Design review of the part built by this model. Coordinates are the model's own, in mm. Face numbers are marked on the shaded views. A direction names the side the tool comes from. Give positions to 0.01 mm unless a question says otherwise; leave off trailing zeros. Write each loop counter-clockwise with the first axis right and the second up, starting at its lowest first coordinate (ties: lowest second). Pieces come first, ordered by that corner, then holes. Notation, with made-up numbers: (78.25, 45.5) -> (134.25, 45.5) arc R22 ccw to (134.25, 77.5) -> close; hole circle Ø5 at (78.5, -19). An arc over 180 degrees is marked (long way). Answer as a JSON object with one key per item and string values.
Autodesk Inventor part; units mm, degrees
ref_plane "YZ Plane" through (0, 0, 0) normal (1, 0, 0) x (0, 1, 0)
ref_plane "XZ Plane" through (0, 0, 0) normal (0, 1, 0) x (-1, 0, 0)
ref_plane "XY Plane" through (0, 0, 0) normal (0, 0, 1) x (1, 0, 0)
sketch "Skizze1" plane through (0, 0, 0) normal (0, 0, 1) x (1, 0, 0)
  circle A0 centre (0, 0) radius 4
  line L0 (2.3094, 4) -> (9.9282, 4)
  line L1 (9.9282, 4) -> (9.9282, -4)
  line L2 (9.9282, -4) -> (6.9282, -4)
  line L3 (6.9282, -4) -> (2.3094, 4)
  line L4 (0, -4) -> (6.9282, -4)
  line L5 (2.3094, 4) -> (0, 4)
  dimension "d0" = 8
  dimension "d2" = 60
  dimension "d10" = 3
extrude "Extrusion1" add sketch "Skizze1" along normal blind 3
extrude "Extrusion2" add sketch "Skizze1" against normal blind 3 contours L3 L0 L1 L2
sketch "Skizze2" plane through (0, 0, 3) normal (0, 0, 1) x (1, 0, 0)
  line L0 (2.3094, 4) -> (9.9282, 4)
  line L1 (9.9282, 4) -> (9.9282, -4)
  line L2 (9.9282, -4) -> (6.9282, -4)
  line L3 (6.9282, -4) -> (2.3094, 4)
  line L4 (6.9282, -4) -> (9.9282, -4)
  line L5 (9.9282, -4) -> (9.9282, 4)
  line L6 (9.9282, 4) -> (6.9282, 4)
  line L7 (6.9282, 4) -> (6.9282, -4)
extrude "Extrusion3" add sketch "Skizze2" along normal blind 6.5 contours L0 L1 L2 L7
mirror "Spiegeln1" about plane through (8.4282, 0, 9.5) normal (0, 0, 1)
sketch "Skizze4" plane through (0, 0, 3) normal (0, 0, 1) x (1, 0, 0)
  line L0 (6.9282, -4) -> (6.9282, 4)
  line L1 (6.9282, 4) -> (0, 4)
  arc A0 (0, 4) -> (0, -4) centre (0, 0) ccw
  line L2 (0, -4) -> (6.9282, -4)
  line L3 (2.3094, 4) -> (9.9282, 4)
  line L4 (9.9282, 4) -> (9.9282, -4)
  line L5 (9.9282, -4) -> (6.9282, -4)
  line L6 (6.9282, -4) -> (2.3094, 4)
  line L7 (-4, 0) -> (-4, -8)
  line L8 (0, 0) -> (0, -8) construction
  line L9 (9.9282, -4) -> (2.773, -10.8828)
  arc A1 (-4, -8) -> (2.773, -10.8828) centre (0, -8) ccw
  arc A2 (0, 4) -> (-4, 0) centre (0, 0) ccw
  line L10 (0, 4) -> (9.9282, 4)
  line L11 (9.9282, -4) -> (9.9282, 4)
  dimension "d18" = 8
extrude "Extrusion4" [suppressed]
extrude "Extrusion5" add sketch "Skizze4" along normal blind 3
sketch "Skizze5" plane through (0, 0, -3) normal (0, 0, -1) x (-1, 0, 0)
  line L0 (-2.3094, 4) -> (-6.9282, -4)
  line L1 (0, -4) -> (-6.9282, -4)
  arc A0 (0, -4) -> (0, 4) centre (0, 0) ccw
  line L2 (-2.3094, 4) -> (0, 4)
  line L3 (0, -4) -> (-9.9282, -4)
  line L4 (-2.773, -10.8828) -> (-9.9282, -4)
  arc A1 (-2.773, -10.8828) -> (4, -8) centre (0, -8) ccw
  line L5 (4, 0) -> (4, -8)
  arc A2 (0, -4) -> (4, 0) centre (0, 0) ccw
hole "Bohrung2" at (0, 0, -3) at (0, -8, -3) direction (0, 0, 1) diameter 3 end through all
sketch "Skizze7" plane through (0, 4, 0) normal (0, 1, 0) x (1, 0, 0)
  line L0 (9.9282, 3) -> (9.9282, -22)
  line L1 (2.3094, 3) -> (9.9282, 3)
  line L2 (0, 0) -> (0, -6)
  line L3 (6.9282, -6) -> (0, -6)
  line L4 (9.9282, 3) -> (16.8306, 3) construction
  line L5 (16.8306, 3) -> (23.047, 0) construction
  spline S0 degree 2 poles (9.9282, 3) (16.8306, 3) (23.047, 0) knots 1 1 1 2 2 2
  arc A0 (24.9282, -9.5) -> (23.047, 0) centre (0, -9.5) ccw
  line L6 (9.9282, -9.5) -> (32.3299, -9.5) construction
  line L7 (23.047, 0) -> (2.3094, 0) construction
  line L8 (9.9282, -22) -> (16.8306, -22) construction
  line L9 (16.8306, -22) -> (23.047, -19) construction
  spline S1 degree 2 poles (9.9282, -22) (16.8306, -22) (23.047, -19) knots 1 1 1 2 2 2
  arc A1 (23.047, -19) -> (24.9282, -9.5) centre (0, -9.5) ccw
  dimension "d30" = 15
extrude "Extrusion6" add sketch "Skizze7" against normal up to surface (8 mm away)
sketch "Skizze8" plane through (0, -4, 16) normal (0, -1, 0) x (1, 0, 0)
  arc A0 (19.9211, -13.9956) -> (20.4401, 0.0137) centre (6.9282, -6.5) ccw
  line L0 (9.9282, -13) -> (9.9282, -10)
  line L1 (0, -16) -> (6.9282, -16)
  line L2 (6.9282, -6.5) -> (21.9282, -6.5)
  line L3 (9.9282, -11.5) -> (21.0703, -11.5)
  arc A1 (23.047, -16) -> (23.047, 3) centre (0, -6.5) ccw
  line L4 (6.9282, -10) -> (6.9282, 0)
  point P0 (15.4993, -1.5)
  point P1 (15.4993, -11.5)
  dimension "d55" = 3
hole "Bohrung3" at (15.4993, -4, 14.5) at (15.4993, -4, 4.5) direction (0, 1, 0) diameter 3 end through all
chamfer "Fase3" distance 1 angle 45 2 edges at (15.4993, 4, 6) (15.4993, 4, 16)
sketch "Skizze12" plane through (0, -4, 0) normal (0, -1, 0) x (1, 0, 0)
  spline S0 degree 2 poles (9.9282, 22) (16.8306, 22) (23.047, 19) knots 0 0 0 1 1 1
  line L0 (9.9282, 22) -> (6.9282, 22)
  line L1 (6.9282, 22) -> (23.047, 19)
extrude "Extrusion10" cut sketch "Skizze12" against normal through all
sketch "Skizze13" plane through (0, -4, 0) normal (0, -1, 0) x (1, 0, 0)
  line L0 (23.047, 19) -> (6.9282, 22)
  line L1 (6.9282, 6) -> (6.9282, 16)
  arc A0 (23.047, 0) -> (23.047, 19) centre (0, 9.5) ccw
  line L2 (23.047, 19) -> (28.3554, 18.012)
  line L3 (23.047, 0) -> (28.3554, 9.2178) construction
  line L4 (28.3554, 9.2178) -> (28.3554, 18.012) construction
  spline S0 degree 2 poles (23.047, 0) (28.3554, 9.2178) (28.3554, 18.012) knots 1 1 1 2 2 2
extrude "Extrusion11" add sketch "Skizze13" against normal up to surface (8 mm away)
fillet "Rundung2" radius 3 4 edges at (23.047, 0, 0) (27.0283, -4, 9.1119) (8.4282, -4, -3) (16.6591, -4, -2.25)
equation "\"d0\" = Finger_diameter"
equation "\"d10\" = FingerWall"
equation "\"d4\" = FingerWall"
equation "\"d6\" = FingerWall"
equation "\"d8\" = -1.5 * FingerWall + 0.5 * Finger_width"
equation "\"d18\" = Finger_diameter"
equation "\"d23\" = bearingHole"
equation "\"FingerLaenge_B\" = 25"
equation "\"Hebel_B\" = 25"
equation "\"Finger_width\" = 22"
equation "\"Finger_diameter\" = 8"
equation "\"FingerWall\" = 3"
equation "\"Hebel_basis_2\" = 15"
equation "\"Join_width\" = 3"
equation "\"bearingHole\" = 3"
equation "\"bearingWall\" = 4"
equation "\"support_D\" = 0.25"
properties part number "FingerTipp"
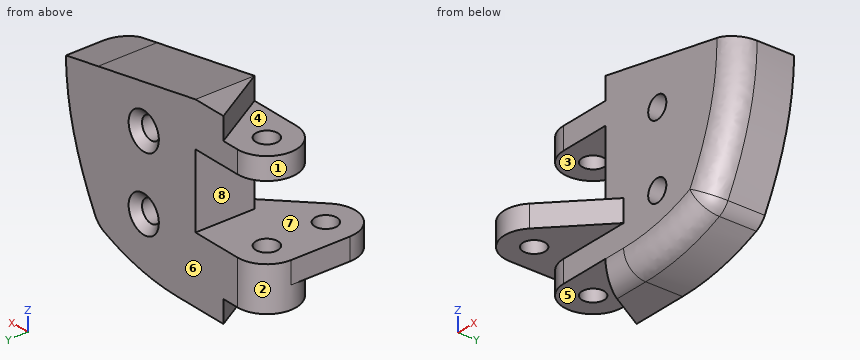
(1) We need section A-A, the plane x = -2. State the section outline as (y, z) points.
Here are the results:
{"outline": "(-11.46, 3) -> (-3.46, 3) -> (-3.46, 0) -> (3.46, 0) -> (3.46, 6) -> (-11.46, 6) -> close; (-3.46, 16) -> (3.46, 16) -> (3.46, 19) -> (-3.46, 19) -> close"}
(2) The part is to be moulded in two halves that separate along Z. For the marked faces 5, 6, 7 and 8, say which applies: +Z half, -Z half, draft (parallel to the pull), parting line (faces both ways), or undercut.
Here are the results:
{"face 5": "-Z half", "face 6": "draft", "face 7": "undercut", "face 8": "undercut"}
(3) We need section C-C, the plane y = -10.25. State the section outline as (x, z) points.
Here are the results:
{"outline": "(-3.31, 3) -> (3.43, 3) -> (3.43, 6) -> (-3.31, 6) -> close"}
(4) For line 1 along Y through (x, z) = (0, 4.85); line 2 along Y through (x, z) = (0, 17.7); line 3 along Z through (x, y) = (-1.5, -1.5), list the stretches that pass through material, from the lowest coordinate up.
Here are the results:
{"line 1": "y = -12 to -9.5, -6.5 to -1.5, 1.5 to 4", "line 2": "y = -4 to -1.5, 1.5 to 4", "line 3": "z = 0 to 6, 16 to 19"}
(5) Clearance check with flat-ended pins moving along their axes: pin 1 (3.5 mm diameter, centred on x = 0, y = -8, fed in from -Z); pin 2 (2.5 mm diameter, centred on x = 1.5, y = 0.5, fed in from -Z); pin 3 (7 mm diameter, centred on x = 1, y = -8, fed in from +Z). State where each tip first meets the part, or that it passes through.
Here are the results:
{"pin 1": "stops at z = 3", "pin 2": "stops at z = 0", "pin 3": "stops at z = 6"}
(6) For the marked faces 1, 2, 3 and 4, list the 3-axis set-ups (+Z, -Z, +X, -X, +Y, -Y) from which the entire face can be reached by the end or side of a thin tool; tool diameter is ignored.
Here are the results:
{"face 1": "+Z, -X", "face 2": "-Z, -X", "face 3": "-X, +Y, -Y", "face 4": "+Z, -X, -Y"}
(7) We need section B-B, the plane y = -2.25. Give the number of separate pieces and of enclosed holes in the cut face, then the cut area to 3 significant figures.
Here are the results:
{"separate pieces": "1", "enclosed holes": "2", "area": "508 mm²"}
(8) We need section D-D, the plane z = 19.5. State the section outline as (x, y) points, then the cut area to 3 significant figures.
Here are the results:
{"outline": "(2.31, 4) -> (6.93, -4) -> (20.36, -4) -> (20.36, 4) -> close", "area": "126 mm²"}
